Design review of the part built by this model. Coordinates are the model's own, in mm. A direction names the side the tool comes from. Give positions to 0.01 mm unless a question says otherwise; leave off trailing zeros. Order: outer loops, then holes, each group sorted by start corner. A loop starts at its lowest first (then second) coordinate and runs counter-clockwise, first axis right, second up. Notation, with made-up numbers: (-17.75, -21) - (4.25, -21) arc R6 cw to (4.25, -14) - close; hole circle Ø2 at (70, -4.75). An arc over 180 degrees is marked (long way). Write each question's results on one line, items separated by ' | '. Start each with the question number.
```python
from build123d import *

# Parameters (mm, degrees)
SKETCH1_W           = 50
SKETCH1_H           = 10
BOSS_EXTRUDE1_DEPTH = 20
CUT_EXTRUDE1_DEPTH  = 70
SKETCH3_3_R         = 3
CUT_EXTRUDE2_DEPTH  = 70
SKETCH4_W           = 5
SKETCH4_H           = 15
CUT_EXTRUDE4_DEPTH  = 20
FILLET5_R           = 2
FILLET6_R           = 2
FILLET7_R           = 2
FILLET8_R           = 2
FILLET9_R           = 2
FILLET10_R          = 2
BOSS_EXTRUDE5_DEPTH = 3
SKETCH14_R          = 1
CUT_EXTRUDE5_DEPTH  = 3


with BuildPart() as part:
    # Sketch1 → Boss-Extrude1 (new body)
    with BuildSketch(Plane(origin=(0, 0, 0), x_dir=(1, 0, 0), z_dir=(0, 1, 0))):
        Rectangle(SKETCH1_W, SKETCH1_H)
    extrude(amount=BOSS_EXTRUDE1_DEPTH)

    # Sketch3 → Cut-Extrude1 (cut)
    with BuildSketch(Plane(origin=(25, 0, 0), x_dir=(0, 0, -1), z_dir=(1, 0, 0))):
        with BuildLine():
            ThreePointArc((0, 20), (2.837274331, 19.286764074), (5, 17.31662479))
            Line((5, 17.31662479), (5, 20))
            Line((5, 20), (0, 20))
        make_face()
        with BuildLine():
            ThreePointArc((-5, 17.31662479), (-2.837274331, 19.286764074), (0, 20))
            Line((0, 20), (-5, 20))
            Line((-5, 20), (-5, 17.31662479))
        make_face()
    extrude(amount=-CUT_EXTRUDE1_DEPTH, mode=Mode.SUBTRACT)

    # Sketch3_3 → Cut-Extrude2 (cut)
    with BuildSketch(Plane(origin=(25, 0, 0), x_dir=(0, 0, -1), z_dir=(1, 0, 0))):
        with Locations((0, 14)):
            Circle(SKETCH3_3_R)
    extrude(amount=-CUT_EXTRUDE2_DEPTH, mode=Mode.SUBTRACT)

    # Sketch4 → Cut-Extrude4 (cut)
    with BuildSketch(Plane.XY.offset(5)):
        with Locations((-12.5, 12.5)):
            Rectangle(SKETCH4_W, SKETCH4_H)
        with Locations((12.5, 12.5)):
            Rectangle(SKETCH4_W, SKETCH4_H)
    extrude(amount=-CUT_EXTRUDE4_DEPTH, mode=Mode.SUBTRACT)

    # Fillet5
    fillet5_edges = [part.edges().sort_by_distance(p)[0] for p in [
        (-20, 17.31662479, 5),
    ]]
    fillet(fillet5_edges, radius=FILLET5_R)

    # Fillet6
    fillet6_edges = [part.edges().sort_by_distance(p)[0] for p in [
        (0, 17.31662479, 5),
    ]]
    fillet(fillet6_edges, radius=FILLET6_R)

    # Fillet7
    fillet7_edges = [part.edges().sort_by_distance(p)[0] for p in [
        (20, 17.31662479, 5),
    ]]
    fillet(fillet7_edges, radius=FILLET7_R)

    # Fillet8
    fillet8_edges = [part.edges().sort_by_distance(p)[0] for p in [
        (20, 17.31662479, -5),
    ]]
    fillet(fillet8_edges, radius=FILLET8_R)

    # Fillet9
    fillet9_edges = [part.edges().sort_by_distance(p)[0] for p in [
        (0, 17.31662479, -5),
    ]]
    fillet(fillet9_edges, radius=FILLET9_R)

    # Fillet10
    fillet10_edges = [part.edges().sort_by_distance(p)[0] for p in [
        (-20, 17.31662479, -5),
    ]]
    fillet(fillet10_edges, radius=FILLET10_R)

    # Sketch13 → Boss-Extrude5 (add)
    with BuildSketch(Plane.XZ):
        with BuildLine():
            Line((-25, 5), (25, 5))
            Line((25, 5), (25, 54))
            ThreePointArc((25, 54), (24.414213562, 55.414213562), (23, 56))
            Line((23, 56), (-23, 56))
            ThreePointArc((-23, 56), (-24.414213562, 55.414213562), (-25, 54))
            Line((-25, 54), (-25, 5))
        make_face()
    extrude(amount=-BOSS_EXTRUDE5_DEPTH)

    # Sketch14 → Cut-Extrude5 (cut)
    with BuildSketch(Plane(origin=(0, 3, 0), x_dir=(1, 0, 0), z_dir=(0, 1, 0))):
        with Locations(Location((-22.45, -13, 0), (0, 0, 270))):
            Circle(SKETCH14_R)
        with Locations(Location((22.45, -13, 0), (0, 0, 270))):
            Circle(SKETCH14_R)
    extrude(amount=-CUT_EXTRUDE5_DEPTH, mode=Mode.SUBTRACT)


solid = part.part
```
Q1. Draft analysis for pull direction X (two halves, no side actions). For faces 4 (the flat face through (-25, 2.5, 15.9)), 5 (the flat face through (25, 2, 13)), 6 (the cylindrical face through (-20.07, 17.343, -4.874)), 7 (the cylindrical face through (-23.34, 1.52, 13.46)), state which applies: pulls with the +X half, pulls with the -X half, needs draft (parallel to the pull), parting line crosses it, or undercut.
Q2. Add section D-D (z = 20.5). Give the boundary of the cut face in (x, y).
Q3. Machinability: for faces 1 (the flat face through (0, 1, 56)), 2 (the flat face through (0, 10, 5)), 3 (the flat face through (15, 10.7, 0.1)), which of the approach directions +Z, -Z, +X, -X, +Y, -Y give a long, thin tool a straight path to every point of the face, cutting with its end or side? Answer none if there is none.
Q4. Add section C-C (y = 14). Give the boundary of the cut face in (x, z).
Q5. Add section B-B (y = 6.5). Give the boundary of the cut face in (x, z).
Q6. Add section A-A (x = 16.5). Give the boundary of the cut face in (y, z).
Q7. For line 1 (X direction, y = 2.3, z = 13); line 2 (Y direction, x = 8, z = 27); line 3 (Z direction, x = 16, y = 8.25), list the stretches that pass through material, from the lowest coordinate up. Write a range as [from, to].
Q8. Insertion check: pin 1 Ø3 at (x, z) = (-14, 18) entering from +Y; pin 2 Ø1.5 at (x, z) = (-12.5, 1.5) entering from +Y; pin 3 Ø12 at (x, z) = (19.5, 10) entering from +Y. Each pin has a flat end and moves straight along its axis. Give the tip position at first contact, or say it passes through.
Verdict:
1) face 4: pulls with the -X half | face 5: pulls with the +X half | face 6: needs draft | face 7: undercut
2) outline: (-25, 0) - (25, 0) - (25, 3) - (-25, 3) - close
3) face 1: +Z, +X, -X, +Y, -Y | face 2: +Z, +X, -X, +Y | face 3: +Z, -Z, +Y
4) outline: (-25, -5) - (-15, -5) - (-15, -3) - (-25, -3) - close; (-25, 3) - (-15, 3) - (-15, 5) - (-25, 5) - close; (-10, -5) - (10, -5) - (10, -3) - (-10, -3) - close; (-10, 3) - (10, 3) - (10, 5) - (-10, 5) - close; (15, -5) - (25, -5) - (25, -3) - (15, -3) - close; (15, 3) - (25, 3) - (25, 5) - (15, 5) - close
5) outline: (-25, -5) - (-15, -5) - (-15, 5) - (-25, 5) - close; (-10, -5) - (10, -5) - (10, 5) - (-10, 5) - close; (15, -5) - (25, -5) - (25, 5) - (15, 5) - close
6) outline: (0, -5) - (16.65, -5) arc R2 ccw to (17.97, -4.5) arc R6 ccw to (17.97, 4.5) arc R2 ccw to (16.65, 5) - (3, 5) - (3, 56) - (0, 56) - close; hole circle Ø6 at (14, 0)
7) line 1: x = [-25, -23.45], [-21.45, 21.45], [23.45, 25] | line 2: y = [0, 3] | line 3: z = [-5, 5]
8) pin 1: stops at y = 3 | pin 2: stops at y = 5 | pin 3: stops at y = 18.47
